```python
from build123d import *

# Parameters (mm, degrees)
BOSS_EXTRUDE4_DEPTH = 12.7
BOSS_EXTRUDE5_DEPTH = 19.05
SKETCH7_W           = 12.7
SKETCH7_H           = 4.7625


with BuildPart() as part:
    # Sketch5 → Boss-Extrude4 (new, symmetric)
    with BuildSketch(Plane.XY):
        Polygon((0, -19.05), (0, 19.05), (-24.490207929, 48.236293283), (-24.490207929, 10.136293283), align=None)
    extrude(amount=BOSS_EXTRUDE4_DEPTH, both=True)

    # Sketch6 → Boss-Extrude5 (add, symmetric)
    with BuildSketch(Plane(origin=(0, 0, 0), x_dir=(1, 0, 0), z_dir=(0, 1, 0))):
        with BuildLine():
            Line((0, 12.7), (0, -12.7))
            ThreePointArc((0, -12.7), (1.051084135, 0), (0, 12.7))
        make_face()
    extrude(amount=BOSS_EXTRUDE5_DEPTH, both=True)

    # Sketch7 → Cut-Revolve5 (revolve, cut)
    with BuildSketch(Plane.XY, mode=Mode.PRIVATE) as cut_revolve5_sk:
        with Locations((-5.298915865, 3.96875)):
            Rectangle(SKETCH7_W, SKETCH7_H)
    revolve(cut_revolve5_sk.sketch.rotate(Axis((-31.455592934, 1.5875, 0), (1, 0, 0)), 180), axis=Axis((-31.455592934, 1.5875, 0), (1, 0, 0)), mode=Mode.SUBTRACT)


solid = part.part
```
Verification items for the finished model (mm, model axes). A direction names the side the tool comes from. Round coordinates to 2 decimals unless told otherwise and drop trailing zeros. Write each loop counter-clockwise with the first axis right and the second up, starting at its lowest first coordinate (ties: lowest second). Pieces come first, ordered by that corner, then holes.
1. Access from +Z, -Z, +X, -X, +Y, -Y to the whole of each face (thin tool, end or side, straight path). Record for faces 5 (the cylindrical face through (-5.21, 6.345, -0.209)), 6 (the flat face through (-12.074, 33.439, 0.178)).
2. Section check C-C on x = -5.25. Enter the section's corners in (y, z) (1 decimal), plus the area to 3 significant figures.
3. Section check D-D on z = -8.75. Enter the section's corners in (x, y), plus the area to 3 significant figures.
4. Scan lines: L1, parallel to Y at x = -1.25, z = -1; L2, parallel to Y at x = -11.5, z = -3.75; L3, parallel to X at y = 12.5, z = 4.75. Record each from-to range of solid material in increasing order.
5. Gauge pin test, flat ends, axial feed: P1, Ø2, axis at y = 22, z = -9, coming from the +X side; P2, Ø12, axis at x = -10.5, z = -7.5, coming from the +Y side; P3, Ø12, axis at x = -7, z = -5, coming from the -Y side. Record the tip position at first contact, or that the pin passes through.
6. Section check B-B on y = 3. Enter the section's corners in (x, z).
7. Draft check along Z on faces 1 (the flat face through (-11.649, 2, 0)), 2 (the flat face through (-24.49, 29, 0)), 3 (the flat face through (-12, 15, 12.7)), 4 (the flat face through (-12, 15, -12.7)). Enter one of: +Z half, -Z half, draft (parallel to the pull), parting line (faces both ways), or undercut.
8. Section check A-A on z = 0. Enter the section's corners in (x, y) (3 decimals), plus the area to 3 significant figures.
Answer:
1. face 5: +X
1. face 6: +Z, -Z, +X, +Y
2. outline: (-12.8, -12.7) - (25.3, -12.7) - (25.3, 12.7) - (-12.8, 12.7) - close; hole circle Ø9.5 at (1.6, 0)
2. area: 896 mm2
3. outline: (-24.49, 10.14) - (0, -19.05) - (0.55, -19.05) - (0.55, 19.05) - (0, 19.05) - (-24.49, 48.24) - close
3. area: 954 mm2
4. L1: y = -17.56 to -3.07, 6.24 to 20.54
4. L2: y = -5.34 to -1.35, 4.52 to 32.76
4. L3: x = -24.49 to 0.9
5. P1: stops at x = -1.64
5. P2: stops at y = 38.71
5. P3: stops at y = -17.86
6. outline: (-18.5, -12.7) - (0, -12.7) arc R77.25 ccw to (0.92, -4.55) - (-11.65, -4.55) - (-11.65, 4.55) - (0.92, 4.55) arc R77.25 ccw to (0, 12.7) - (-18.5, 12.7) - close
7. face 1: undercut
7. face 2: draft
7. face 3: +Z half
7. face 4: -Z half
8. outline: (-24.49, 10.136) - (0, -19.05) - (1.051, -19.05) - (1.051, -3.175) - (-11.649, -3.175) - (-11.649, 6.35) - (1.051, 6.35) - (1.051, 19.05) - (0, 19.05) - (-24.49, 48.236) - close
8. area: 852 mm2
